Verification items for the finished model (mm, model axes). Face numbers are marked on the shaded views. A direction names the side the tool comes from. Give positions to 0.01 mm unless a question says otherwise; leave off trailing zeros. Write each loop counter-clockwise with the first axis right and the second up, starting at its lowest first coordinate (ties: lowest second). Pieces come first, ordered by that corner, then holes.
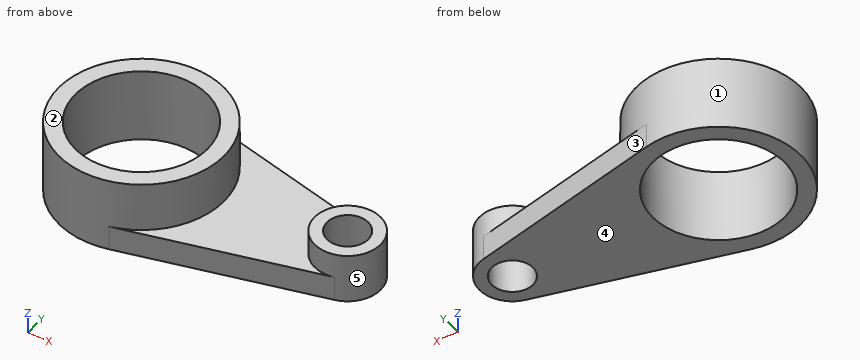
Autodesk Fusion 360 part; units mm, degrees
sketch "스케치1" plane through (0, 0, 0) normal (0, 0, 1) x (1, 0, 0)
  circle A0 centre (0, 0) radius 50
  circle A1 centre (125.1784, 0) radius 20
  line L0 (11.9829, 48.5429) -> (129.9716, 19.4171)
  line L1 (11.9829, -48.5429) -> (129.9716, -19.4171)
  circle A2 centre (0, 0) radius 40
  circle A3 centre (125.1784, 0) radius 12.5
  dimension "d1" = 100
  dimension "d2" = 40
  dimension "d3" = 80
  dimension "d4" = 25
extrude "돌출4" add sketch "스케치1" along normal blind 45 contours A0 makes body 1
extrude "돌출5" add sketch "스케치1" along normal blind 30 separate body contours A1 makes body 2
extrude "돌출6" add sketch "스케치1" along normal blind 15 contours A0 A1 L0 L1 bodies 1 2
Item 1: Set-up check for the marked faces 1 and 2: record each of +Z, -Z, +X, -X, +Y, -Y from which the full face is reachable in a straight line by a thin tool's end or side.
Answer key:
face 1: +Z
face 2: +Z, +X, -X, +Y, -Y
Item 2: Sectioned sample at B-B on z = 26.5. Record the cut outline in (x, y).
Answer key:
outline: circle Ø100 at (0, 0); circle Ø40 at (125.18, 0); hole circle Ø80 at (0, 0); hole circle Ø25 at (125.18, 0)
Item 3: Sectioned sample at D-D on z = 42. Record the cut outline in (x, y).
Answer key:
outline: circle Ø100 at (0, 0); hole circle Ø80 at (0, 0)
Item 4: Sectioned sample at C-C on x = 0. Record the cut outline in (y, z), then the cut area to 3 significant figures.
Answer key:
outline: (-50, 0) - (-40, 0) - (-40, 45) - (-50, 45) - close; (40, 0) - (50, 0) - (50, 45) - (40, 45) - close
area: 900 mm2
Item 5: Sectioned sample at A-A on y = 0. Record the cut outline in (x, z).
Answer key:
outline: (-50, 0) - (-40, 0) - (-40, 45) - (-50, 45) - close; (40, 0) - (112.68, 0) - (112.68, 30) - (105.18, 30) - (105.18, 15) - (50, 15) - (50, 45) - (40, 45) - close; (137.68, 0) - (145.18, 0) - (145.18, 30) - (137.68, 30) - close
Item 6: Release check for a two-part mould opening along X. For the marked faces 3, 4 and 5 record: released by +X, released by -X, zero draft, split by the parting line, or undercut.
Answer key:
face 3: released by +X
face 4: zero draft
face 5: undercut
Item 7: Depth check by flat-ended pin: pin 1 (12 mm diameter, centred on x = -19.5, z = 30.5, fed in from +Y); pin 2 (2 mm diameter, centred on x = 26, z = 36, fed in from +Y); pin 3 (4 mm diameter, centred on y = 36, z = 10.5, fed in from -X). Enter the tip coordinate at first touch or a pass-through.
Answer key:
pin 1: stops at y = 48.14
pin 2: stops at y = 43.3
pin 3: stops at x = -36.66
Item 8: Scan lines: line 1 along Y through (x, z) = (0, 27.5); line 2 along X through (y, z) = (35.5, 37); line 3 along Y through (x, z) = (16, 31.5). Record each from-to range of solid material in increasing order.
Answer key:
line 1: y = -50 to -40, 40 to 50
line 2: x = -35.21 to -18.43, 18.43 to 35.21
line 3: y = -47.37 to -36.66, 36.66 to 47.37
